```python
from build123d import *

# Parameters (mm, degrees)
SKETCH1_W                = 25
SKETCH1_H                = 22
BOSS_EXTRUDE1_DEPTH      = 10
SKETCH2_R                = 3
CUT_EXTRUDE1_DEPTH       = 30.086079144
CHAMFER1_SIZE            = 1
BOSS_EXTRUDE4_DEPTH      = 10
BOSS_EXTRUDE4_DEPTH_BACK = 10
SKETCH3_W                = 25
SKETCH3_H                = 8
SKETCH10_W               = 1
SKETCH10_H               = 1.5
CUT_EXTRUDE6_DEPTH       = 6
SKETCH5_W                = 25
SKETCH5_H                = 10
BOSS_EXTRUDE3_DEPTH      = 40
SKETCH6_R                = 11
CUT_EXTRUDE3_DEPTH       = 8
SKETCH7_R                = 3
SKETCH7_R_2              = 1.5
CUT_EXTRUDE4_DEPTH       = 8
SKETCH8_R                = 3
CUT_EXTRUDE5_DEPTH       = 5
FILLET1_R                = 5


with BuildPart() as part:
    # Sketch1 → Boss-Extrude1 (new body)
    with BuildSketch(Plane(origin=(0, 0, 0), x_dir=(1, 0, 0), z_dir=(0, 1, 0))):
        Rectangle(SKETCH1_W, SKETCH1_H)
    extrude(amount=BOSS_EXTRUDE1_DEPTH)

    # Sketch2 → Cut-Extrude1 (cut, through all)
    with BuildSketch(Plane(origin=(12.5, 0, 0), x_dir=(0, 0, -1), z_dir=(1, 0, 0))):
        with Locations((-6, 5)):
            Circle(SKETCH2_R)
        with Locations((6, 5)):
            Circle(SKETCH2_R)
    extrude(amount=-CUT_EXTRUDE1_DEPTH, mode=Mode.SUBTRACT)

    # Chamfer1
    chamfer1_edges = [part.edges().sort_by_distance(p)[0] for p in [
        (-12.5, 5, 9),
        (12.5, 5, 9),
        (-12.5, 5, -3),
        (12.5, 5, -3),
    ]]
    chamfer(chamfer1_edges, length=CHAMFER1_SIZE)

    # Sketch3 → Boss-Extrude4 (add, two sides: drawn at the far end of the back side and taken through both)
    with BuildSketch(Plane(origin=(0, 10, 0), x_dir=(1, 0, 0), z_dir=(0, 1, 0)).offset(-BOSS_EXTRUDE4_DEPTH_BACK)):
        with Locations((0, 15)):
            Rectangle(SKETCH3_W, SKETCH3_H)
    extrude(amount=BOSS_EXTRUDE4_DEPTH + BOSS_EXTRUDE4_DEPTH_BACK)

    # Sketch10 → Cut-Extrude6 (cut)
    with BuildSketch(Plane(origin=(0, 18, 0), x_dir=(1, 0, 0), z_dir=(0, 1, 0))):
        with Locations((12, 17.75)):
            Rectangle(SKETCH10_W, SKETCH10_H)
        with Locations((10, 17.75)):
            Rectangle(SKETCH10_W, SKETCH10_H)
        Polygon((12.5, 19), (-12.5, 19), (-12.5, 18.5), (-11.5, 18.5), (-10.5, 18.5), (-9.5, 18.5), (-8.5, 18.5), (-7.5, 18.5), (-6.5, 18.5), (-5.5, 18.5), (-4.5, 18.5), (-3.5, 18.5), (-2.5, 18.5), (-1.5, 18.5), (-0.5, 18.5), (0.5, 18.5), (1.5, 18.5), (2.5, 18.5), (3.5, 18.5), (4.5, 18.5), (5.5, 18.5), (6.5, 18.5), (7.5, 18.5), (8.5, 18.5), (9.5, 18.5), (10.5, 18.5), (11.5, 18.5), (12.5, 18.5), align=None)
        with Locations((8, 17.75)):
            Rectangle(SKETCH10_W, SKETCH10_H)
        with Locations((6, 17.75)):
            Rectangle(SKETCH10_W, SKETCH10_H)
        with Locations((4, 17.75)):
            Rectangle(SKETCH10_W, SKETCH10_H)
        with Locations((2, 17.75)):
            Rectangle(SKETCH10_W, SKETCH10_H)
        with Locations((0, 17.75)):
            Rectangle(SKETCH10_W, SKETCH10_H)
        with Locations((-2, 17.75)):
            Rectangle(SKETCH10_W, SKETCH10_H)
        with Locations((-4, 17.75)):
            Rectangle(SKETCH10_W, SKETCH10_H)
        with Locations((-6, 17.75)):
            Rectangle(SKETCH10_W, SKETCH10_H)
        with Locations((-8, 17.75)):
            Rectangle(SKETCH10_W, SKETCH10_H)
        with Locations((-10, 17.75)):
            Rectangle(SKETCH10_W, SKETCH10_H)
        with Locations((-12, 17.75)):
            Rectangle(SKETCH10_W, SKETCH10_H)
    extrude(amount=-CUT_EXTRUDE6_DEPTH, mode=Mode.SUBTRACT)

    # Sketch5 → Boss-Extrude3 (add)
    with BuildSketch(Plane.XY.offset(11)):
        with Locations((0, 5)):
            Rectangle(SKETCH5_W, SKETCH5_H)
    extrude(amount=BOSS_EXTRUDE3_DEPTH)

    # Sketch6 → Cut-Extrude3 (cut)
    with BuildSketch(Plane.XZ):
        with Locations(Location((0, 35, 0), (0, 0, 270))):
            Circle(SKETCH6_R)
    extrude(amount=-CUT_EXTRUDE3_DEPTH, mode=Mode.SUBTRACT)

    # Sketch7 → Cut-Extrude4 (cut)
    with BuildSketch(Plane.XZ.offset(-8)):
        with Locations(Location((0, 35, 0), (0, 0, 270))):
            Circle(SKETCH7_R)
        with Locations(Location((-6, 35, 0), (0, 0, 270))):
            Circle(SKETCH7_R_2)
        with Locations(Location((6, 35, 0), (0, 0, 270))):
            Circle(SKETCH7_R_2)
    extrude(amount=-CUT_EXTRUDE4_DEPTH, mode=Mode.SUBTRACT)

    # Sketch8 → Cut-Extrude5 (cut)
    with BuildSketch(Plane.XY.offset(51)):
        with Locations((6, 5)):
            Circle(SKETCH8_R)
        with Locations((-6, 5)):
            Circle(SKETCH8_R)
    extrude(amount=-CUT_EXTRUDE5_DEPTH, mode=Mode.SUBTRACT)

    # Fillet1
    fillet1_edges = [part.edges().sort_by_distance(p)[0] for p in [
        (0, 20, -11),
    ]]
    fillet(fillet1_edges, radius=FILLET1_R)


solid = part.part
```
Geometry check sheet. Reference: the model listing, model coordinates, mm. A direction names the side the tool comes from. Give positions to 0.01 mm unless a question says otherwise; leave off trailing zeros. Loops run counter-clockwise (first coordinate to the right, second up) from the corner with the lowest first, then second, coordinate; pieces in that order, holes last. Notation, with made-up numbers: (32.25, -30) - (41.25, -30) arc R13 cw to (41.25, -25) - close; hole circle Ø6 at (27.5, 86). An arc over 180 degrees is marked (long way). Use CSV: the item, a comma, the result in double quotes. Start each with the question number.
Q1. Access from +Z, -Z, +X, -X, +Y, -Y to the whole of each face (thin tool, end or side, straight path). Record for faces 1 (the face through (-7.5, 15, -18)), 2 (the face through (0, 12, -11)), 3 (the face through (6, 5, 46)), 4 (the face through (0, 9, 38)).
Q2. Section check A-A, the plane y = 5. Count the separate pieces of the cut face and the enclosed holes in it, and give its area (3 significant figures).
Q3. Section check B-B, the plane z = 35. Record the cut outline in (x, y).
Q4. Scan lines: probe 1 along X at (y, z) = (9.05, 35); probe 2 along Z at (x, y) = (-5, 3.25); probe 3 along Z at (x, y) = (7.5, 6.75). Record each from-to range of solid material in increasing order. Write a range as from..to.
Q5. Release check for a two-part mould opening along X. For faces 5 (the face through (-11.5, 15, -18)), 6 (the face through (-6.9, 9, 36.2)), 7 (the face through (0, 6, -19)) record: +X half, -X half, draft (parallel to the pull), parting line (faces both ways), or undercut.
Q6. Go/stop test with flat-tipped pins: pin 1 Ø1.1 at (x, y) = (-2, 15) entering from -Z; pin 2 Ø5 at (x, z) = (-6, 35) entering from -Y; pin 3 Ø5.5 at (y, z) = (5, 6) entering from -X; pin 4 Ø3 at (x, y) = (2.5, 16) entering from +Z. Record where each tip stops, or that it passes through.
Q7. Section check C-C, the plane z = -6. Record the cut outline in (x, y), and give its area (3 significant figures).
Findings below:
1,face 1,"-Z"
1,face 2,"+Z, +X, -X, +Y"
1,face 3,"+Z"
1,face 4,"+Y, -Y"
2,separate pieces,"3"
2,enclosed holes,"1"
2,area,"1,010 mm^2"
3,outline,"(-12.5, 0) - (-11, 0) - (-11, 8) - (-7.5, 8) - (-7.5, 10) - (-12.5, 10) - close; (-4.5, 8) - (-3, 8) - (-3, 10) - (-4.5, 10) - close; (3, 8) - (4.5, 8) - (4.5, 10) - (3, 10) - close; (7.5, 8) - (11, 8) - (11, 0) - (12.5, 0) - (12.5, 10) - (7.5, 10) - close"
4,probe 1,"x = -12.5..-7.5, -4.5..-3, 3..4.5, 7.5..12.5"
4,probe 2,"z = -19..-8.44, -3.56..3.56, 8.44..25.2, 44.8..46"
4,probe 3,"z = -19..-8.44, -3.56..3.56, 8.44..26.95, 43.05..46"
5,face 5,"-X half"
5,face 6,"undercut"
5,face 7,"draft"
6,pin 1,"stops at z = -18.5"
6,pin 2,"stops at y = 8"
6,pin 3,"passes through"
6,pin 4,"stops at z = -11"
7,outline,"(-12.5, 0) - (12.5, 0) - (12.5, 1) - (11.5, 2) - (-11.5, 2) - (-12.5, 1) - close; (-12.5, 9) - (-11.5, 8) - (11.5, 8) - (12.5, 9) - (12.5, 10) - (-12.5, 10) - close"
7,area,"98.0 mm^2"
